from build123d import *

# Parameters (mm, degrees)
BOSS_EXTRUDE1_DEPTH      = 1
SKETCH2_R                = 1.325
CUT_EXTRUDE1_DEPTH       = 2
SKETCH3_R                = 0.5
CUT_EXTRUDE2_DEPTH       = 2
LPATTERN1_COUNT          = 20
LPATTERN1_PITCH          = 2.54
BOSS_EXTRUDE6_DEPTH      = 0.4
BOSS_EXTRUDE6_DEPTH_BACK = 4.5
CUT_EXTRUDE9_DEPTH       = 5.25
SKETCH_1_W               = 4.7
SKETCH_1_H               = 2.3
EXTRUDE_1_DEPTH          = 2
SKETCH_2_W               = 1.86
SKETCH_2_H               = 1
EXTRUDE_2_DEPTH          = 1
SKETCH_9_R               = 2.75
SKETCH_9_R_2             = 1.325
EXTRUDE_8_DEPTH          = 1.5
SKETCH_10_R              = 1.05
EXTRUDE_9_DEPTH          = 2.5
SKETCH_11_R              = 0.5
EXTRUDE_10_DEPTH         = 3
SKETCH_12_R              = 7
EXTRUDE_11_DEPTH         = 2
SKETCH_13_W              = 1
SKETCH_13_H              = 2
EXTRUDE_12_DEPTH         = 0.5
FILLET_1_R               = 0.5
EXTRUDE_13_DEPTH         = 1


with BuildPart() as part:
    # Sketch1 → Boss-Extrude1 (new body)
    with BuildSketch(Plane(origin=(0, 0, 0), x_dir=(1, 0, 0), z_dir=(0, 1, 0))):
        with BuildLine():
            Line((-28.75, 15), (28.75, 15))
            ThreePointArc((28.75, 15), (31.401650429, 13.901650429), (32.5, 11.25))
            Line((32.5, 11.25), (32.5, -11.25))
            ThreePointArc((32.5, -11.25), (31.401650429, -13.901650429), (28.75, -15))
            Line((28.75, -15), (-28.75, -15))
            ThreePointArc((-28.75, -15), (-31.401650429, -13.901650429), (-32.5, -11.25))
            Line((-32.5, -11.25), (-32.5, 11.25))
            ThreePointArc((-32.5, 11.25), (-31.401650429, 13.901650429), (-28.75, 15))
        make_face()
    extrude(amount=BOSS_EXTRUDE1_DEPTH)

    # Sketch2 → Cut-Extrude1 (cut, through all)
    with BuildSketch(Plane(origin=(0, 1, 0), x_dir=(1, 0, 0), z_dir=(0, 1, 0))):
        with Locations((-29.025, 11.525)):
            Circle(SKETCH2_R)
        with Locations((29.025, 11.525)):
            Circle(SKETCH2_R)
        with Locations((29.025, -11.525)):
            Circle(SKETCH2_R)
        with Locations((-29.025, -11.525)):
            Circle(SKETCH2_R)
    extrude(amount=-CUT_EXTRUDE1_DEPTH, mode=Mode.SUBTRACT)

    # Sketch3 → Cut-Extrude2 (cut, through all)
    with BuildSketch(Plane(origin=(0, 1, 0), x_dir=(1, 0, 0), z_dir=(0, 1, 0))):
        with Locations((-24.128, 13)):
            Circle(SKETCH3_R)
        with Locations((-24.128, 10.5)):
            Circle(SKETCH3_R)
    cut_extrude2 = extrude(amount=-CUT_EXTRUDE2_DEPTH, mode=Mode.SUBTRACT)

    # LPattern1: Cut-Extrude2 ×20
    with Locations(*[(i * LPATTERN1_PITCH, 0, 0) for i in range(1, LPATTERN1_COUNT)]):
        add(cut_extrude2, mode=Mode.SUBTRACT)

    # Sketch15 → Boss-Extrude6 (add, two sides)
    with BuildSketch(Plane.XY.offset(15)) as boss_extrude6_sk:
        with BuildLine():
            Line((-24, 4), (-17, 4))
            ThreePointArc((-17, 4), (-16.292893219, 3.707106781), (-16, 3))
            Line((-16, 3), (-16, 2))
            ThreePointArc((-16, 2), (-16.292893219, 1.292893219), (-17, 1))
            Line((-17, 1), (-24, 1))
            ThreePointArc((-24, 1), (-24.707106781, 1.292893219), (-25, 2))
            Line((-25, 2), (-25, 3))
            ThreePointArc((-25, 3), (-24.707106781, 3.707106781), (-24, 4))
        make_face()
    extrude(amount=BOSS_EXTRUDE6_DEPTH)
    extrude(boss_extrude6_sk.sketch, amount=-BOSS_EXTRUDE6_DEPTH_BACK)

    # Sketch16 → Cut-Extrude9 (cut)
    with BuildSketch(Plane.XY.offset(15.4)):
        with BuildLine():
            Line((-17, 3.68), (-24, 3.68))
            ThreePointArc((-24, 3.68), (-24.480832611, 3.480832611), (-24.68, 3))
            Line((-24.68, 3), (-24.68, 2))
            ThreePointArc((-24.68, 2), (-24.480832611, 1.519167389), (-24, 1.32))
            Line((-24, 1.32), (-17, 1.32))
            ThreePointArc((-17, 1.32), (-16.519167389, 1.519167389), (-16.32, 2))
            Line((-16.32, 2), (-16.32, 3))
            ThreePointArc((-16.32, 3), (-16.519167389, 3.480832611), (-17, 3.68))
        make_face()
    extrude(amount=-CUT_EXTRUDE9_DEPTH, mode=Mode.SUBTRACT)

    # 草图1 → 凸台-拉伸1 (add)
    with BuildSketch(Plane(origin=(0, 1, 0), x_dir=(1, 0, 0), z_dir=(0, 1, 0))):
        with Locations((-10.52, -13.05)):
            Rectangle(SKETCH_1_W, SKETCH_1_H)
        with Locations((21.95, -13.05)):
            Rectangle(SKETCH_1_W, SKETCH_1_H)
    extrude(amount=EXTRUDE_1_DEPTH)

    # 草图2 → 凸台-拉伸2 (add)
    with BuildSketch(Plane.XY.offset(14.2)):
        with Locations((-10.52, 2)):
            Rectangle(SKETCH_2_W, SKETCH_2_H)
        with Locations((21.95, 2)):
            Rectangle(SKETCH_2_W, SKETCH_2_H)
    extrude(amount=EXTRUDE_2_DEPTH)

    # 草图9 → 凸台-拉伸8 (add)
    with BuildSketch(Plane.XZ):
        with Locations((29.025, 11.525)):
            Circle(SKETCH_9_R)
        with Locations((29.025, 11.525)):
            Circle(SKETCH_9_R_2, mode=Mode.SUBTRACT)
        with Locations((29.025, -11.525)):
            Circle(SKETCH_9_R)
        with Locations((29.025, -11.525)):
            Circle(SKETCH_9_R_2, mode=Mode.SUBTRACT)
        with Locations((-29.025, 11.525)):
            Circle(SKETCH_9_R)
        with Locations((-29.025, 11.525)):
            Circle(SKETCH_9_R_2, mode=Mode.SUBTRACT)
        with Locations((-29.025, -11.525)):
            Circle(SKETCH_9_R)
        with Locations((-29.025, -11.525)):
            Circle(SKETCH_9_R_2, mode=Mode.SUBTRACT)
    extrude(amount=EXTRUDE_8_DEPTH)

    # 草图10 → 凸台-拉伸9 (add)
    with BuildSketch(Plane(origin=(0, 1, 0), x_dir=(1, 0, 0), z_dir=(0, 1, 0))):
        with Locations((24.132, 13)):
            Circle(SKETCH_10_R)
        with Locations((21.592, 13)):
            Circle(SKETCH_10_R)
        with Locations((19.052, 13)):
            Circle(SKETCH_10_R)
        with Locations((21.592, 10.5)):
            Circle(SKETCH_10_R)
        with Locations((19.052, 10.5)):
            Circle(SKETCH_10_R)
        with Locations((-24.128, 10.5)):
            Circle(SKETCH_10_R)
        with Locations((13.972, 10.5)):
            Circle(SKETCH_10_R)
    extrude(amount=EXTRUDE_9_DEPTH)

    # 草图11 → 凸台-拉伸10 (add)
    with BuildSketch(Plane.XZ.offset(-1)):
        with Locations((24.132, -13)):
            Circle(SKETCH_11_R)
        with Locations((21.592, -13)):
            Circle(SKETCH_11_R)
        with Locations((21.592, -10.5)):
            Circle(SKETCH_11_R)
        with Locations((19.052, -10.5)):
            Circle(SKETCH_11_R)
        with Locations((19.052, -13)):
            Circle(SKETCH_11_R)
        with Locations((-24.128, -10.5)):
            Circle(SKETCH_11_R)
    extrude(amount=EXTRUDE_10_DEPTH)

    # 草图12 → 凸台-拉伸11 (add)
    with BuildSketch(Plane(origin=(0, 1, 0), x_dir=(1, 0, 0), z_dir=(0, 1, 0))):
        with Locations((12.5, 0)):
            Circle(SKETCH_12_R)
    extrude(amount=EXTRUDE_11_DEPTH)

    # 草图13 → 凸台-拉伸12 (add)
    with BuildSketch(Plane(origin=(0, 1, 0), x_dir=(1, 0, 0), z_dir=(0, 1, 0))):
        with Locations((17.6, -13)):
            Rectangle(SKETCH_13_W, SKETCH_13_H)
        with Locations((15.4, -13)):
            Rectangle(SKETCH_13_W, SKETCH_13_H)
        with Locations((13.2, -13)):
            Rectangle(SKETCH_13_W, SKETCH_13_H)
        with Locations((11, -13)):
            Rectangle(SKETCH_13_W, SKETCH_13_H)
    extrude(amount=EXTRUDE_12_DEPTH)

    # 圆角1
    fillet_1_edges = [part.edges().sort_by_distance(p)[0] for p in [
        (5.5, 3, 0),
    ]]
    fillet(fillet_1_edges, radius=FILLET_1_R)

    # 草图14 → 凸台-拉伸13 (add)
    with BuildSketch(Plane(origin=(0, 0, 10.5), x_dir=(-1, 0, 0), z_dir=(0, 0, -1))):
        with BuildLine():
            Line((16, 3), (16, 2))
            ThreePointArc((16, 2), (16.292893219, 1.292893219), (17, 1))
            Line((17, 1), (24, 1))
            ThreePointArc((24, 1), (24.707106781, 1.292893219), (25, 2))
            Line((25, 2), (25, 3))
            ThreePointArc((25, 3), (24.707106781, 3.707106781), (24, 4))
            Line((24, 4), (17, 4))
            ThreePointArc((17, 4), (16.292893219, 3.707106781), (16, 3))
        make_face()
    extrude(amount=-EXTRUDE_13_DEPTH)


solid = part.part
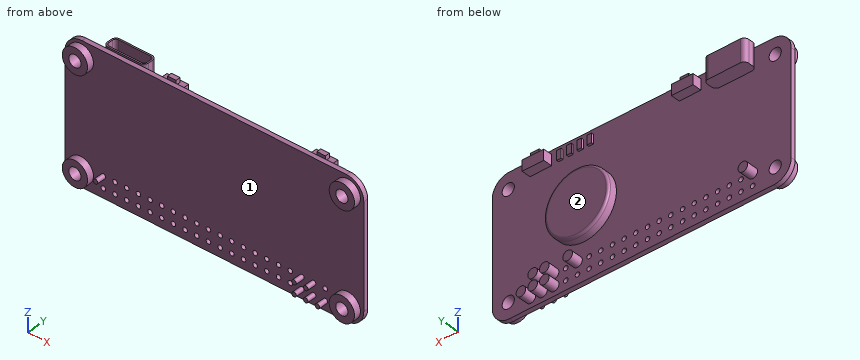
Read the model definition and answer for the solid it produces. Units are mm, in the model's axes. Face numbers are marked on the shaded views. Coordinates: 2 decimals unless noted, no trailing zeros. Loops run counter-clockwise (first coordinate to the right, second up) from the corner with the lowest first, then second, coordinate; pieces in that order, holes last.
Q1. The mould has two halves that part along Z. Classify the marked faces 1 and 2: +Z half, -Z half, draft (parallel to the pull), parting line (faces both ways), or undercut.
Q2. Consider probe 1 along Y at (x, z) = (-6.5, 2.5); probe 2 along Z at (x, y) = (-24, 1.75); probe 3 along Z at (x, y) = (18.5, 3.45). Determine where each line is inside the solid, lowest interval first.
Q3. The part is cut by section B-B on z = -8. Write down the section's boundary in (x, y), and give its area (3 significant figures).
Q4. Each of these flat-tipped pins is pushed along its axis until it touches: pin 1 Ø1.2 at (x, y) = (-22.5, 2.5) entering from +Z; pin 2 Ø6 at (x, z) = (-16, 5.5) entering from -Y; pin 3 Ø1.5 at (y, z) = (2.5, 4.5) entering from -X. Where does it stop, or does it pass through?
Q5. The part is cut by section A-A on z = 0. Write down the section's boundary in (x, y).
Results below:
1. face 1: undercut
1. face 2: draft
2. probe 1: y = 0 to 1
2. probe 2: z = -11.54 to -9.46, 10.5 to 11.5
2. probe 3: z = -13.89 to -12.11, -11.39 to -9.61
3. outline: (-32.5, 0) - (32.5, 0) - (32.5, 1) - (-32.5, 1) - close
3. area: 65.0 mm2
4. pin 1: stops at z = 11.5
4. pin 2: stops at y = 0
4. pin 3: stops at x = 6.59
5. outline: (-32.5, 0) - (32.5, 0) - (32.5, 1) - (19.5, 1) - (19.5, 2.5) arc R0.5 ccw to (19, 3) - (6, 3) arc R0.5 ccw to (5.5, 2.5) - (5.5, 1) - (-32.5, 1) - close
